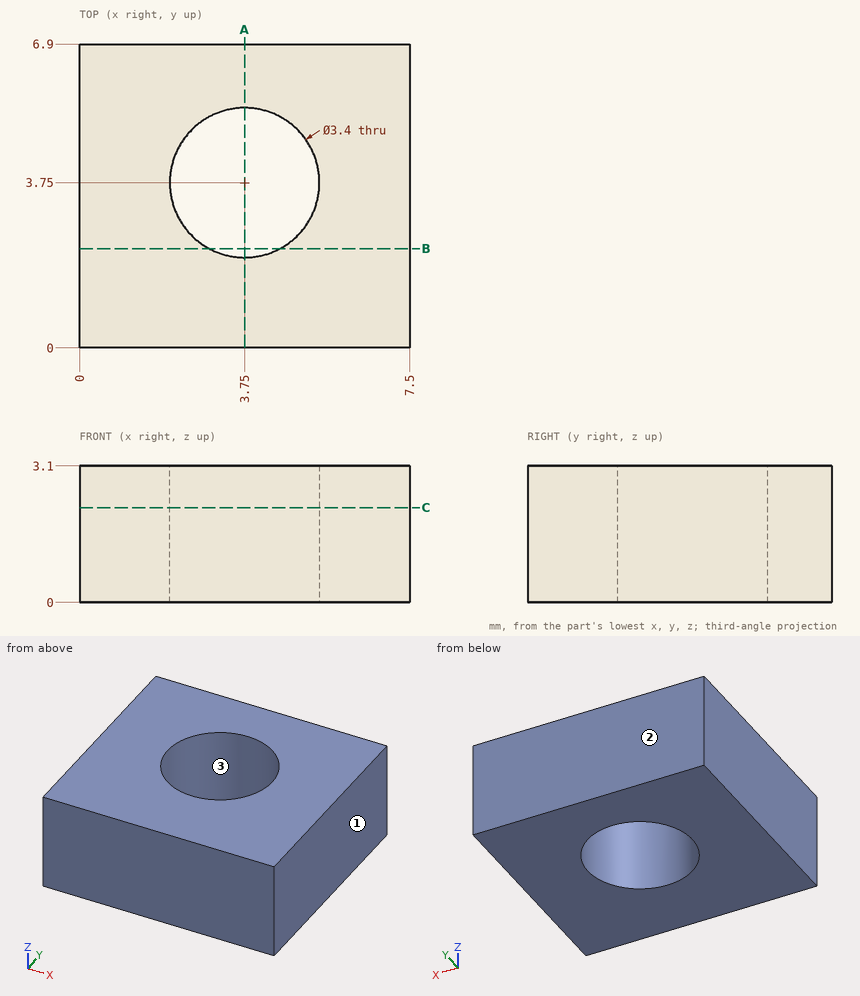
Geometry: see drawing. Coordinates: mm, zero at the bounding-box minimum. Give positions to 0.01 mm unless a question says otherwise; leave off trailing zeros. Loops run counter-clockwise (first coordinate to the right, second up) from the corner with the lowest first, then second, coordinate; pieces in that order, holes last. Notation, with made-up numbers: (12.25, 16.5) - (70.25, 16.5) arc R14 cw to (70.25, 39.5) - close; hole circle Ø7 at (-21.75, 61). An arc over 180 degrees is marked (long way). Use CSV: the item, a comma, the result in double quotes.
1) Cut plane C-C (z = 2.15). Output: boundary loops of the cut face in (x, y).
Worked out:
outline,"(0, 0) - (7.5, 0) - (7.5, 6.9) - (0, 6.9) - close; hole circle Ø3.4 at (3.75, 3.75)"
2) Cut plane B-B (y = 2.25). Output: boundary loops of the cut face in (x, z), and give its area (3 significant figures).
Worked out:
outline,"(0, 0) - (2.95, 0) - (2.95, 3.1) - (0, 3.1) - close; (4.55, 0) - (7.5, 0) - (7.5, 3.1) - (4.55, 3.1) - close"
area,"18.3 mm^2"
3) Mould query, pull axis Y, two halves, no side actions, for the marked faces 1, 2 and 3. Classes: +Y half, -Y half, draft (parallel to the pull), parting line (faces both ways), or undercut.
Worked out:
face 1,"draft"
face 2,"+Y half"
face 3,"undercut"
4) Line query: line 1 (Y direction, x = 3.75, z = 1.4); line 2 (Y direction, x = 3, z = 0.7); line 3 (X direction, y = 4.5, z = 2.7). Output: solid intervals per line, ascending.
Worked out:
line 1,"y = 0 to 2.05, 5.45 to 6.9"
line 2,"y = 0 to 2.22, 5.28 to 6.9"
line 3,"x = 0 to 2.22, 5.28 to 7.5"
5) Cut plane A-A (x = 3.75). Output: boundary loops of the cut face in (y, z), and give its area (4 significant figures).
Worked out:
outline,"(0, 0) - (2.05, 0) - (2.05, 3.1) - (0, 3.1) - close; (5.45, 0) - (6.9, 0) - (6.9, 3.1) - (5.45, 3.1) - close"
area,"10.85 mm^2"
